from build123d import *

# Parameters (mm, degrees)
SKETCH1_W                                         = 127
SKETCH1_H                                         = 25.4
SKETCH1_R                                         = 4.7625
BOSS_EXTRUDE1_DEPTH                               = 6.35
CSK_FOR_6_FLAT_HEAD_MACHINE_SCREW_100_D           = 3.7973
CSK_FOR_6_FLAT_HEAD_MACHINE_SCREW_100_CSINK_D     = 7.0866
CSK_FOR_6_FLAT_HEAD_MACHINE_SCREW_100_CSINK_ANGLE = 100
SKETCH5_W                                         = 6.35
SKETCH5_H                                         = 22.225
CUT_EXTRUDE1_DEPTH                                = 103.587389576
SKETCH6_W                                         = 6.35
SKETCH6_H                                         = 1.5875
CUT_EXTRUDE2_DEPTH                                = 103.587389576
TAP_DRILL_FOR_6_32_TAP1_D                         = 2.7051
TAP_DRILL_FOR_6_32_TAP1_DEPTH                     = 6.35
TAP_DRILL_FOR_6_32_TAP1_TIP                       = 0.81269403


with BuildPart() as part:
    # Sketch1 → Boss-Extrude1 (new body)
    with BuildSketch(Plane.XY):
        with Locations((-38.1, 0)):
            Rectangle(SKETCH1_W, SKETCH1_H)
        Polygon((-88.9, 8.193180488), (-62.954928456, 0), (-88.9, -8.193180488), align=None, mode=Mode.SUBTRACT)
        Polygon((-84.682571544, -9.525), (-58.7375, -1.331819512), (-32.792428456, -9.525), align=None, mode=Mode.SUBTRACT)
        Polygon((-28.575, -8.193180488), (-54.520071544, 0), (-28.575, 8.193180488), align=None, mode=Mode.SUBTRACT)
        Polygon((-32.792428456, 9.525), (-58.7375, 1.331819512), (-84.682571544, 9.525), align=None, mode=Mode.SUBTRACT)
        Circle(SKETCH1_R, mode=Mode.SUBTRACT)
    extrude(amount=BOSS_EXTRUDE1_DEPTH)

    # CSK for #6 Flat Head Machine Screw (100)1 (through all)
    with Locations(Plane(origin=(0, 0, 0), x_dir=(-1, 0, 0), z_dir=(0, 0, -1))):
        with Locations((-22.225, 4.7625), (-22.225, -4.7625), (22.225, 0)):
            CounterSinkHole(CSK_FOR_6_FLAT_HEAD_MACHINE_SCREW_100_D / 2, CSK_FOR_6_FLAT_HEAD_MACHINE_SCREW_100_CSINK_D / 2, counter_sink_angle=CSK_FOR_6_FLAT_HEAD_MACHINE_SCREW_100_CSINK_ANGLE)

    # Sketch5 → Cut-Extrude1 (cut, through all)
    with BuildSketch(Plane(origin=(0, 0, 0), x_dir=(-1, 0, 0), z_dir=(0, 0, -1))):
        with Locations((98.425, 0)):
            Rectangle(SKETCH5_W, SKETCH5_H)
    extrude(amount=-CUT_EXTRUDE1_DEPTH, mode=Mode.SUBTRACT)

    # Sketch6 → Cut-Extrude2 (cut, through all)
    with BuildSketch(Plane(origin=(0, 0, 0), x_dir=(-1, 0, 0), z_dir=(0, 0, -1))):
        with Locations((22.225, 11.90625)):
            Rectangle(SKETCH6_W, SKETCH6_H)
        with Locations((-22.225, 11.90625)):
            Rectangle(SKETCH6_W, SKETCH6_H)
    cut_extrude2 = extrude(amount=-CUT_EXTRUDE2_DEPTH, mode=Mode.SUBTRACT)

    # Mirror3: Cut-Extrude2 across plane
    add(cut_extrude2.mirror(Plane(origin=(0, 0, 0), x_dir=(0, 0, 1), z_dir=(0, -1, 0))), mode=Mode.SUBTRACT)

    # Tap Drill for #6-32 Tap1
    with Locations(Plane.ZY.offset(95.25)):
        with Locations((3.175, 4.7625), (3.175, -4.7625)):
            Hole(TAP_DRILL_FOR_6_32_TAP1_D / 2, depth=TAP_DRILL_FOR_6_32_TAP1_DEPTH)
            with Locations((0, 0, -(TAP_DRILL_FOR_6_32_TAP1_DEPTH + TAP_DRILL_FOR_6_32_TAP1_TIP / 2))):  # 118° drill point
                Cone(0, TAP_DRILL_FOR_6_32_TAP1_D / 2, TAP_DRILL_FOR_6_32_TAP1_TIP, mode=Mode.SUBTRACT)


solid = part.part
The listing builds one solid part. Answer for the finished solid, in the listing's coordinates (mm). A direction names the side the tool comes from. Coordinates: 2 decimals unless noted, no trailing zeros. Loops run counter-clockwise (first coordinate to the right, second up) from the corner with the lowest first, then second, coordinate; pieces in that order, holes last. Notation, with made-up numbers: M -39,62 L -16,62 A21 ccw -16,92 Z; hole C 15,-15 d7. An arc over 180 degrees is marked long. Answer in a Markdown table with one row per item.
1) Determine the mould class of faces 1 (the flat face through (-41.73, 4.04, 3.13)), 2 (the flat face through (-64, 12.7, 3)), 3 (the flat face through (-22, 11.112, 3)), 4 (the flat face through (-95.25, 0, 3)) for opening direction X: released by +X, released by -X, zero draft, split by the parting line, or undercut.
Answers below:
| item | result |
|---|---|
| face 1 | undercut |
| face 2 | zero draft |
| face 3 | undercut |
| face 4 | released by -X |
2) Which of the six approach directions +Z, -Z, +X, -X, +Y, -Y give full straight-line access (tool end or side, diameter ignored) to faces 5 (the flat face through (-98, -11.112, 3)), 6 (the cylindrical face through (-92.031, 4.822, 4.526)), 7 (the flat face through (-45.95, -5.37, 3.13))?
Answers below:
| item | result |
|---|---|
| face 5 | +Z, -Z, -X |
| face 6 | -X |
| face 7 | +Z, -Z |
3) Find section B-B (x = -81.5). Determine the outline of the cut face in (y, z) (3 decimals), then the cut area to 3 significant figures.
Answers below:
| item | result |
|---|---|
| outline | M -12.7,0 L -9.525,0 L -9.525,6.35 L -12.7,6.35 Z; M -8.52,0 L -5.856,0 L -5.856,6.35 L -8.52,6.35 Z; M 5.856,0 L 8.52,0 L 8.52,6.35 L 5.856,6.35 Z; M 9.525,0 L 12.7,0 L 12.7,6.35 L 9.525,6.35 Z |
| area | 74.2 mm^2 |
4) Find section C-C (x = -31.5). Determine the outline of the cut face in (y, z), then the cut area to 3 significant figures.
Answers below:
| item | result |
|---|---|
| outline | M -12.7,0 L -7.27,0 L -7.27,6.35 L -12.7,6.35 Z; M 7.27,0 L 12.7,0 L 12.7,6.35 L 7.27,6.35 Z |
| area | 69.0 mm^2 |
5) Find section A-A (x = 0). Determine the outline of the cut face in (y, z).
Answers below:
| item | result |
|---|---|
| outline | M -12.7,0 L -4.76,0 L -4.76,6.35 L -12.7,6.35 Z; M 4.76,0 L 12.7,0 L 12.7,6.35 L 4.76,6.35 Z |
6) Given pin 1 (1 mm diameter, centred on y = 1.5, z = 0.5, fed in from -X); pin 2 (3 mm diameter, centred on x = -16, y = -5.5, fed in from -Z); pin 3 (0.8 mm diameter, centred on y = 12, z = 4, fed in from +X), each flat-ended and moving along its own axis, determine where each tip first touches the part or whether it passes through.
Answers below:
| item | result |
|---|---|
| pin 1 | x = -95.25 |
| pin 2 | z = 0 |
| pin 3 | x = 19.05 |
7) Find the intervals of material crossed by probe 1 along X at (y, z) = (11.25, 1.75); probe 2 along Y at (x, z) = (-73, 5.25) (3 decimals); probe 3 along Y at (x, z) = (-95, 2.25), in increasing order.
Answers below:
| item | result |
|---|---|
| probe 1 | -101.6 to -25.4, -19.05 to 19.05 |
| probe 2 | -12.7 to -9.525, -5.836 to -3.172, 3.172 to 5.836, 9.525 to 12.7 |
| probe 3 | -12.7 to -5.75, -3.78 to 3.78, 5.75 to 12.7 |
